from build123d import *

# Parameters (mm, degrees)
F1_DEPTH    = 76.2
F2_R        = 3.175
F3_DEPTH    = 3.175
F4_T1_DEPTH = 76.2
F4_T3_DEPTH = 92.075


# Not quite as in the source:
# - a fillet or chamfer that OpenCascade refuses, or shapes differently, is made with other operations: its cross-section is extruded or revolved along the edge and cut away or added


with BuildPart() as f1:
    # F0 (on Top) → F1 (new body)
    with BuildSketch(Plane.XY):
        Polygon((-34.0479501394, 7.7857396193), (-37.2229501394, 7.7857396193), (-37.2229501394, -17.6142603807), (-11.8229501394, -17.6142603807), (-11.8229501394, -14.4392603807), (-34.0479501394, -14.4392603807), align=None)
    extrude(amount=F1_DEPTH)

    # F2 (on face) → F3 (cut)
    with BuildSketch(Plane(origin=(0, -14.4392603807, 0), x_dir=(-1, 0, 0), z_dir=(0, 1, 0))):
        with Locations((21.3479501394, 63.5)):
            Circle(F2_R)
        with Locations((21.3479501394, 12.7)):
            Circle(F2_R)
    extrude(amount=-F3_DEPTH, mode=Mode.SUBTRACT)

    # F4: fillet of radius 3.175 on 4 edges, made by hand

    # F4_s2 → F4_t1 (join)
    with BuildSketch(Plane.XY):
        with BuildLine():
            add(Edge.make_bspline(
                [(-34.0479501394, -11.2642603807), (-34.0479501394, -14.4392603807), (-30.8729501394, -14.4392603807)],
                knots=[0, 0, 0, 1, 1, 1], degree=2, weights=[1, 1, 1]))
            Line((-30.8729501394, -14.4392603807), (-34.0479501394, -14.4392603807))
            Line((-34.0479501394, -14.4392603807), (-34.0479501394, -11.2642603807))
        make_face()
    extrude(amount=F4_T1_DEPTH)

    # F4_s4 → F4_t3 (cut)
    with BuildSketch(Plane.XY.offset(-7.9375)):
        with BuildLine():
            add(Edge.make_bspline(
                [(-11.8229501394, -17.6142603807), (-11.8229501394, -14.4392603807), (-14.9979501394, -14.4392603807)],
                knots=[0, 0, 0, 1, 1, 1], degree=2, weights=[1, 1, 1]))
            Line((-14.9979501394, -14.4392603807), (-11.8229501394, -14.4392603807))
            Line((-11.8229501394, -14.4392603807), (-11.8229501394, -17.6142603807))
        make_face()
        with BuildLine():
            add(Edge.make_bspline(
                [(-34.0479501394, 4.6107396193), (-34.0479501394, 7.7857396193), (-37.2229501394, 7.7857396193)],
                knots=[0, 0, 0, 1, 1, 1], degree=2, weights=[1, 1, 1]))
            Line((-37.2229501394, 7.7857396193), (-34.0479501394, 7.7857396193))
            Line((-34.0479501394, 7.7857396193), (-34.0479501394, 4.6107396193))
        make_face()
        with BuildLine():
            add(Edge.make_bspline(
                [(-37.2229501394, -14.4392603807), (-37.2229501394, -17.6142603807), (-34.0479501394, -17.6142603807)],
                knots=[0, 0, 0, 1, 1, 1], degree=2, weights=[1, 1, 1]))
            Line((-34.0479501394, -17.6142603807), (-37.2229501394, -17.6142603807))
            Line((-37.2229501394, -17.6142603807), (-37.2229501394, -14.4392603807))
        make_face()
    extrude(amount=F4_T3_DEPTH, mode=Mode.SUBTRACT)


solid = f1.part
Design review of the part built by this model. Coordinates are the model's own, in mm. A direction names the side the tool comes from. Give positions to 0.01 mm unless a question says otherwise; leave off trailing zeros. Loops run counter-clockwise (first coordinate to the right, second up) from the corner with the lowest first, then second, coordinate; pieces in that order, holes last. Notation, with made-up numbers: M 68.25,58.5 L 77.25,58.5 A9 cw 77.25,70.5 Z; hole C 2.25,74.25 d5. An arc over 180 degrees is marked long. One line per question, with ' | ' between items. Start each with the question number.
1. For faces 4 (the face through (-34.048, -3, 38)), 5 (the face through (-23, -17.614, 38)), list the 3-axis set-ups (+Z, -Z, +X, -X, +Y, -Y) from which the entire face can be reached by the end or side of a thin tool; tool diameter is ignored.
2. Add section B-B (y = 2.5). Write out the cut boundary in (x, z).
3. To check wall thickness, follow L1, parallel to Y at x = -16.75, z = 14.5; L2, parallel to X at y = 1.25, z = 72; L3, parallel to X at y = 5.75, z = 17.5. State the ranges of each line that lie inside material, in increasing order.
4. The part is to be moulded in two halves that separate along Z. For faces 1 (the face through (-20.66, -16, 9.6)), 2 (the face through (-23, -14.439, 38)), 3 (the face through (-30, -15, 76.2)), say which applies: released by +Z, released by -Z, zero draft, split by the parting line, or undercut.
5. Insertion check: P1, Ø12.5, axis at y = -0.5, z = 43, coming from the +X side; P2, Ø1.5, axis at x = -24.5, z = 31, coming from the +Y side. Each pin has a flat end and moves straight along its axis. Give the tip position at first contact, or say it passes through.
6. Add section A-A (x = -25.5). Write out the cut boundary in (y, z), plus the area to 3 significant figures.
Worked out:
1) face 4: +Z, -Z, +X, +Y | face 5: +Z, -Z, +X, -X, -Y
2) outline: M -37.22,0 L -34.05,0 L -34.05,76.2 L -37.22,76.2 Z
3) L1: y = -17.61 to -14.44 | L2: x = -37.22 to -34.05 | L3: x = -37.22 to -34.17
4) face 1: undercut | face 2: zero draft | face 3: released by +Z
5) P1: stops at x = -34.05 | P2: stops at y = -14.44
6) outline: M -17.61,0 L -14.44,0 L -14.44,76.2 L -17.61,76.2 Z | area: 242 mm²
